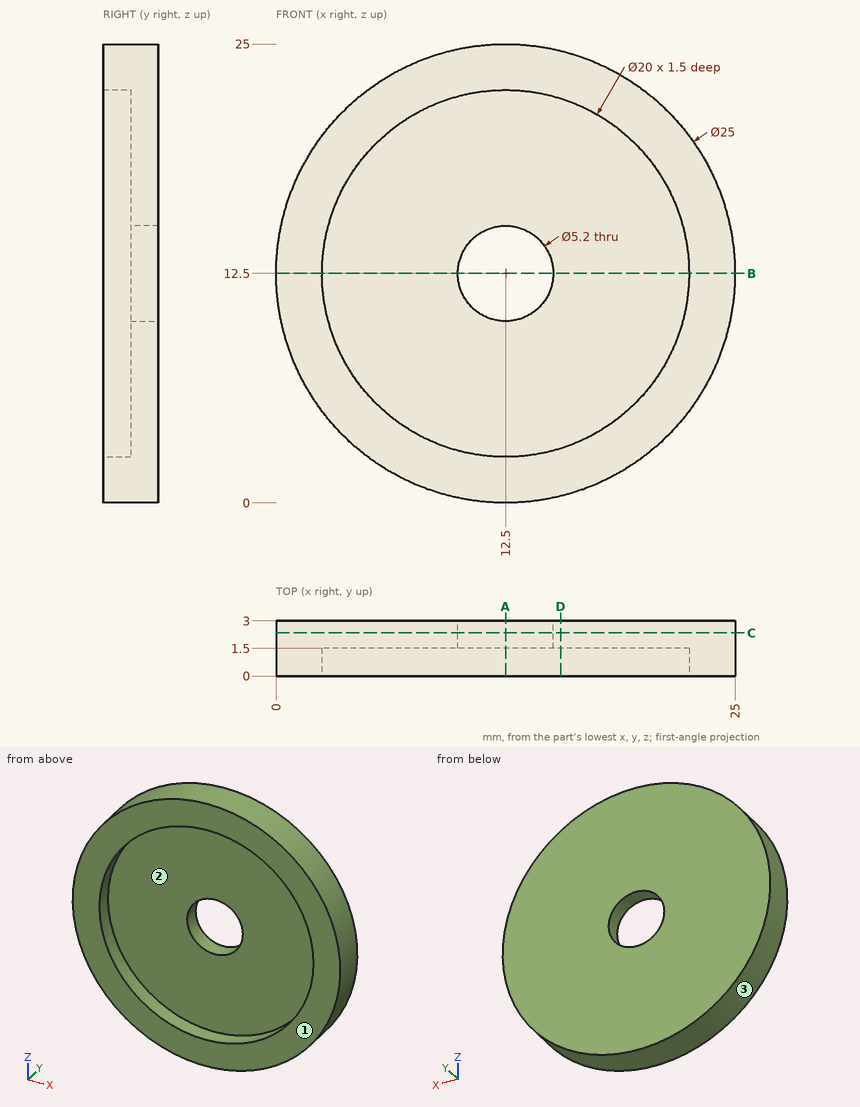
Job drawing, mm, ordinate dimensions from the low corner. One solid piece. Coordinates: 2 decimals unless noted, no trailing zeros. Order: outer loops, then holes, each group sorted by start corner. A loop starts at its lowest first (then second) coordinate and runs counter-clockwise, first axis right, second up. Notation, with made-up numbers: (82.25, 59.25) - (122.25, 59.25) arc R21 cw to (122.25, 92.25) - close; hole circle Ø2 at (-35, 87). An arc over 180 degrees is marked (long way). Return JSON: item names as keys, results as strings. Group by question number.
1) Saw through at C-C, the plane y = 2.35. Write the cut outline in (x, z), plus the area to 3 significant figures.
2) Saw through at D-D, the plane x = 15.5. Write the cut outline in (y, z).
3) Saw through at A-A, the plane x = 12.5. Write the cut outline in (y, z).
4) Probe line 1 (X direction, y = 0.5, z = 12.5); line 2 (X direction, y = 2.7, z = 12.5); line 3 (Y direction, x = 15.5, z = 13.25). List the from-to ranges inside material, lowest first. Write a range as from..to.
5) Saw through at B-B, the plane z = 12.5. Write the cut outline in (x, y).
6) Flat gauge pins, fed straight in: P1, Ø1.5, axis at x = 3, z = 8, coming from the -Y side; P2, Ø8, axis at x = 13, z = 7, coming from the -Y side; P3, Ø1.5, axis at x = 4, y = 2, coming from the +Z side. Where does each tip first touch, or does it go through?
7) Mould opens along X. For the marked faces 1, 2 and 3 say: released by +X, released by -X, zero draft, split by the parting line, or undercut.
Values found:
{
 "1": {"outline": "circle Ø25 at (12.5, 12.5); hole circle Ø5.2 at (12.5, 12.5)", "area": "470 mm²"},
 "2": {"outline": "(0, 0.37) - (3, 0.37) - (3, 24.63) - (0, 24.63) - (0, 22.04) - (1.5, 22.04) - (1.5, 2.96) - (0, 2.96) - close"},
 "3": {"outline": "(0, 0) - (3, 0) - (3, 9.9) - (1.5, 9.9) - (1.5, 2.5) - (0, 2.5) - close; (0, 22.5) - (1.5, 22.5) - (1.5, 15.1) - (3, 15.1) - (3, 25) - (0, 25) - close"},
 "4": {"line 1": "x = 0..2.5, 22.5..25", "line 2": "x = 0..9.9, 15.1..25", "line 3": "y = 1.5..3"},
 "5": {"outline": "(0, 0) - (2.5, 0) - (2.5, 1.5) - (9.9, 1.5) - (9.9, 3) - (0, 3) - close; (15.1, 1.5) - (22.5, 1.5) - (22.5, 0) - (25, 0) - (25, 3) - (15.1, 3) - close"},
 "6": {"P1": "stops at y = 0", "P2": "stops at y = 1.5", "P3": "stops at z = 22.31"},
 "7": {"face 1": "zero draft", "face 2": "undercut", "face 3": "split by the parting line"}
}
